Here's how the part is built. I have some questions about the finished solid (model axes, mm). A direction names the side the tool comes from. Give positions to 0.01 mm unless a question says otherwise; leave off trailing zeros. Write each loop counter-clockwise with the first axis right and the second up, starting at its lowest first coordinate (ties: lowest second). Pieces come first, ordered by that corner, then holes. Notation, with made-up numbers: (62.5, 40.25) -> (66.5, 40.25) arc R25 cw to (66.5, 63.25) -> close; hole circle Ø7 at (66.25, 40.5). An arc over 180 degrees is marked (long way). Use CSV: the item, a comma, the result in double quotes. Start each with the question number.
(1) Suppose I cut it at C-C on x = 1.5. List the corners of the cut face in (y, z) for me, plus the area to 3 significant figures.
(2) Suppose I cut it at A-A on z = 81. List the corners of the cut face in (x, y) for me.
(3) Suppose I cut it at B-B on y = 11.25. List the corners of the cut face in (x, z) for me, plus the area to 3 significant figures.
(4) I need wall thicknesses on L1, parallel to Z at x = 0.6, y = 5; L2, parallel to Z at x = 2.75, y = 8.5; L3, parallel to Z at x = 1.1, y = 11.75. Which ranges of each line are inside material? Lowest first, please. Write a range as [from, to].
(5) Which directions (+Z, -Z, +X, -X, +Y, -Y) give clear straight access to the entire face, cutting with the end or side of a thin tool? Please do faces 1 (the flat face through (1, 0, 20)), 2 (the flat face through (1, 3, 65.467)), 3 (the flat face through (1, 9.993, 82)), 4 (the flat face through (1, 12, 76.56)), 5 (the flat face through (1, 5.632, 16)).
(6) If we mould it in two halves opening along Y, with no side actions, what happens to faces 6 (the flat face through (1, -4.409, 76)), 7 (the flat face through (1, 18.364, 61)), 8 (the flat face through (1, 5, 39.785)), 9 (the flat face through (1, 12, 80.165))? For each: pulls with the +Y half, pulls with the -Y half, needs draft (parallel to the pull), parting line crosses it, or undercut.
(7) For pin 1 Ø1.5 at (x, y) = (1, 4) entering from -Z; pin 2 Ø1.5 at (x, z) = (1, 82.5) entering from +Y; pin 3 Ø0.8 at (x, y) = (1, 20) entering from +Z; pin 4 Ø1.5 at (x, z) = (1, 14.5) entering from -Y, each with a flat end and sliding along its axis, tell me the tip position at first contact or that it passes through.
(8) Suppose I cut it at D-D on y = -0.75. List the corners of the cut face in (x, z) for me, plus the area to 3 significant figures.
from build123d import *

# Parameters (mm, degrees)
F1_DEPTH = 3


with BuildPart() as f1:
    # F0 (on Right) → F1 (new body)
    with BuildSketch(Plane.YZ):
        Polygon((0, 39.784912), (0, 0), (5.631864, 0), (5.631864, 33.050187), (21.127917, 33.050187), (21.127917, 36.418896), (18.364444, 36.418896), (18.364444, 86.97556), (13.37989, 86.97556), (13.37989, 83.370075), (9.992642, 83.370075), (9.992642, 80.1652), (13.37989, 80.1652), (13.37989, 76.559722), (9.992642, 76.559722), (9.992642, 70.550583), (5.986553, 70.550583), (5.986553, 76.559722), (0, 76.559722), (0, 80.1652), (5.986553, 80.1652), (5.986553, 83.370075), (0, 83.370075), (0, 87.072618), (-4.40907, 87.072618), (-4.40907, 65.46703), (9.992642, 65.46703), (9.992642, 39.784912), align=None)
    extrude(amount=F1_DEPTH)


solid = f1.part
Geometry says:
1,outline,"(-4.41, 65.47) -> (9.99, 65.47) -> (9.99, 39.78) -> (0, 39.78) -> (0, 0) -> (5.63, 0) -> (5.63, 33.05) -> (21.13, 33.05) -> (21.13, 36.42) -> (18.36, 36.42) -> (18.36, 86.98) -> (13.38, 86.98) -> (13.38, 83.37) -> (9.99, 83.37) -> (9.99, 80.17) -> (13.38, 80.17) -> (13.38, 76.56) -> (9.99, 76.56) -> (9.99, 70.55) -> (5.99, 70.55) -> (5.99, 76.56) -> (0, 76.56) -> (0, 80.17) -> (5.99, 80.17) -> (5.99, 83.37) -> (0, 83.37) -> (0, 87.07) -> (-4.41, 87.07) -> close"
1,area,"891 mm²"
2,outline,"(0, -4.41) -> (3, -4.41) -> (3, 5.99) -> (0, 5.99) -> close; (0, 9.99) -> (3, 9.99) -> (3, 18.36) -> (0, 18.36) -> close"
3,outline,"(0, 33.05) -> (3, 33.05) -> (3, 76.56) -> (0, 76.56) -> close; (0, 80.17) -> (3, 80.17) -> (3, 83.37) -> (0, 83.37) -> close"
3,area,"140 mm²"
4,L1,"[0, 39.78], [65.47, 76.56], [80.17, 83.37]"
4,L2,"[33.05, 39.78], [65.47, 70.55]"
4,L3,"[33.05, 76.56], [80.17, 83.37]"
5,face 1,"-Z, +X, -X, -Y"
5,face 2,"+X, -X, -Y"
5,face 3,"+Z, +X, -X"
5,face 4,"+X, -X"
5,face 5,"-Z, +X, -X, +Y"
6,face 6,"pulls with the -Y half"
6,face 7,"pulls with the +Y half"
6,face 8,"needs draft"
6,face 9,"undercut"
7,pin 1,"z = 0"
7,pin 2,"y = 18.36"
7,pin 3,"z = 36.42"
7,pin 4,"y = 0"
8,outline,"(0, 65.47) -> (3, 65.47) -> (3, 87.07) -> (0, 87.07) -> close"
8,area,"64.8 mm²"
